Read the model definition and answer for the solid it produces. Units are mm, in the model's axes. Give positions to 0.01 mm unless a question says otherwise; leave off trailing zeros. Order: outer loops, then holes, each group sorted by start corner. A loop starts at its lowest first (then second) coordinate and runs counter-clockwise, first axis right, second up. Notation, with made-up numbers: (-26, 73.5) -> (-6, 73.5) arc R28 ccw to (-6, 108.5) -> close; hole circle Ø2 at (84.25, 84). An arc over 180 degrees is marked (long way). Use one line per item in the form item = value.
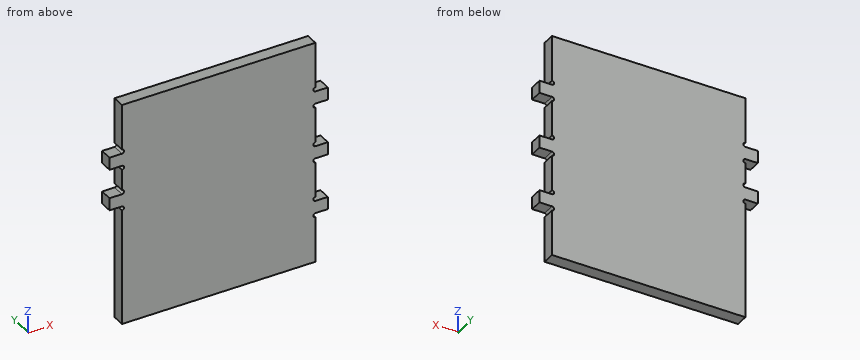
```python
from build123d import *

# Parameters (mm, degrees)
BOSS_EXTRUDE1_DEPTH     = 19.05
CUT_EXTRUDE1_DEPTH      = 466.557212515
CUT_EXTRUDE1_DEPTH_BACK = 466.557212515


with BuildPart() as part:
    # Sketch1 → Boss-Extrude1 (new body)
    with BuildSketch(Plane(origin=(0, 0, 0), x_dir=(1, 0, 0), z_dir=(0, 1, 0))):
        Polygon((0, 0), (295.275, 0), (295.275, 76.2), (314.325, 76.2), (314.325, 95.25), (295.275, 95.25), (295.275, 161.925), (314.325, 161.925), (314.325, 180.975), (295.275, 180.975), (295.275, 247.65), (314.325, 247.65), (314.325, 266.7), (295.275, 266.7), (295.275, 342.9), (0, 342.9), (0, 158.75), (-19.05, 158.75), (-19.05, 139.7), (0, 139.7), (0, 95.25), (-19.05, 95.25), (-19.05, 76.2), (0, 76.2), align=None)
    extrude(amount=BOSS_EXTRUDE1_DEPTH)

    # Sketch2 → Cut-Extrude1 (cut, two sides: drawn at the far end of the back side and taken through both)
    with BuildSketch(Plane(origin=(0, 19.05, 0), x_dir=(1, 0, 0), z_dir=(0, 1, 0)).offset(-CUT_EXTRUDE1_DEPTH_BACK)):
        with BuildLine():
            Line((0, 165.1), (0, 158.75))
            ThreePointArc((0, 158.75), (3.175, 161.925), (0, 165.1))
        make_face()
        with BuildLine():
            Line((0, 139.7), (0, 133.35))
            ThreePointArc((0, 133.35), (3.175, 136.525), (0, 139.7))
        make_face()
        with BuildLine():
            Line((0, 101.6), (0, 95.25))
            ThreePointArc((0, 95.25), (3.175, 98.425), (0, 101.6))
        make_face()
        with BuildLine():
            Line((0, 76.2), (0, 69.85))
            ThreePointArc((0, 69.85), (3.175, 73.025), (0, 76.2))
        make_face()
        with BuildLine():
            Line((295.275, 273.05), (295.275, 266.7))
            ThreePointArc((295.275, 266.7), (292.1, 269.875), (295.275, 273.05))
        make_face()
        with BuildLine():
            Line((295.275, 241.3), (295.275, 247.65))
            ThreePointArc((295.275, 247.65), (292.1, 244.475), (295.275, 241.3))
        make_face()
        with BuildLine():
            Line((295.275, 101.6), (295.275, 95.25))
            ThreePointArc((295.275, 95.25), (292.1, 98.425), (295.275, 101.6))
        make_face()
        with BuildLine():
            Line((295.275, 76.2), (295.275, 69.85))
            ThreePointArc((295.275, 69.85), (292.1, 73.025), (295.275, 76.2))
        make_face()
        with BuildLine():
            Line((295.275, 161.925), (295.275, 155.575))
            ThreePointArc((295.275, 155.575), (292.1, 158.75), (295.275, 161.925))
        make_face()
        with BuildLine():
            Line((295.275, 187.325), (295.275, 180.975))
            ThreePointArc((295.275, 180.975), (292.1, 184.15), (295.275, 187.325))
        make_face()
    extrude(amount=CUT_EXTRUDE1_DEPTH + CUT_EXTRUDE1_DEPTH_BACK, mode=Mode.SUBTRACT)


solid = part.part
```
Item 1: Straight lines are drawn through the part: L1, parallel to Z at x = 296, y = 14 (3 decimals); L2, parallel to X at y = 7.5, z = -219 (3 decimals); L3, parallel to X at y = 18, z = -136.5 (3 decimals). For each, find the intervals that lie inside material, in ascending order. Write a range as from..to.
Checks:
L1 = -266.7..-247.65, -180.975..-161.925, -95.25..-76.2
L2 = 0..295.275
L3 = 3.175..295.275
Item 2: The part is cut by section B-B on z = -314. Give the vertices of the cut face in (x, y) (3 decimals), and give its area (4 significant figures).
Checks:
outline = (0, 0) -> (295.275, 0) -> (295.275, 19.05) -> (0, 19.05) -> close
area = 5,625 mm²
Item 3: Given pin 1 Ø5.5 at (x, y) = (-9.5, 8.5) entering from +Z; pin 2 Ø5.5 at (y, z) = (7.5, -220) entering from +X (3 decimals); pin 3 Ø9.5 at (x, y) = (-5.5, 7) entering from -Z, each flat-ended and moving along its own axis, determine where each tip first touches the part or whether it passes through.
Checks:
pin_1 = -76.2
pin_2 = 295.275
pin_3 = -158.75
